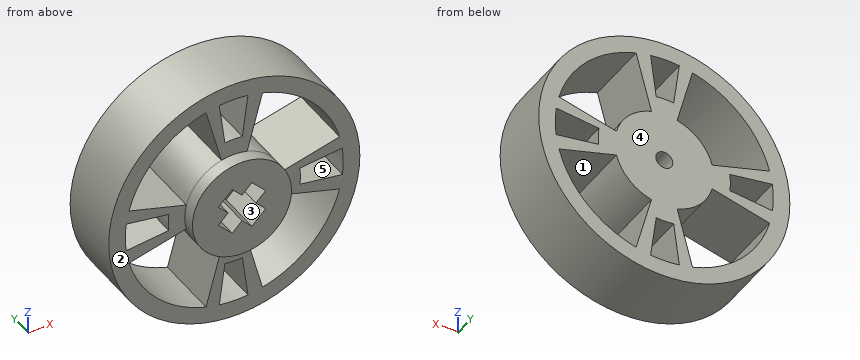
from build123d import *

# Parameters (mm, degrees)
SKETCH1_R           = 9.525
BOSS_EXTRUDE1_DEPTH = 2.54
SKETCH3_R           = 24.13
BOSS_EXTRUDE2_DEPTH = 12.7
CUT_EXTRUDE2_DEPTH  = 16.24
CUT_EXTRUDE3_DEPTH  = 8.466666667
SKETCH5_R           = 1.63195
CUT_EXTRUDE4_DEPTH  = 16.24


with BuildPart() as part:
    # Sketch1 → Boss-Extrude1 (new body)
    with BuildSketch(Plane(origin=(0, 0, 0), x_dir=(1, 0, 0), z_dir=(0, 1, 0))):
        Circle(SKETCH1_R)
    extrude(amount=BOSS_EXTRUDE1_DEPTH)

    # Sketch3 → Boss-Extrude2 (add)
    with BuildSketch(Plane(origin=(0, 2.54, 0), x_dir=(1, 0, 0), z_dir=(0, 1, 0))):
        Circle(SKETCH3_R)
        with BuildLine():
            Line((-2.465251405, 9.200443495), (-5.42355309, 20.24097569))
            ThreePointArc((-5.42355309, 20.24097569), (-14.8174226, 14.8174226), (-20.24097569, 5.42355309))
            Line((-20.24097569, 5.42355309), (-9.200443495, 2.465251405))
            ThreePointArc((-9.200443495, 2.465251405), (-6.735192091, 6.735192091), (-2.465251405, 9.200443495))
        make_face(mode=Mode.SUBTRACT)
        with BuildLine():
            Line((9.200443495, 2.465251405), (20.24097569, 5.42355309))
            ThreePointArc((20.24097569, 5.42355309), (14.8174226, 14.8174226), (5.42355309, 20.24097569))
            Line((5.42355309, 20.24097569), (2.465251405, 9.200443495))
            ThreePointArc((2.465251405, 9.200443495), (6.735192091, 6.735192091), (9.200443495, 2.465251405))
        make_face(mode=Mode.SUBTRACT)
        with BuildLine():
            Line((9.200443495, -2.465251405), (20.24097569, -5.42355309))
            ThreePointArc((20.24097569, -5.42355309), (14.8174226, -14.8174226), (5.42355309, -20.24097569))
            Line((5.42355309, -20.24097569), (2.465251405, -9.200443495))
            ThreePointArc((2.465251405, -9.200443495), (6.735192091, -6.735192091), (9.200443495, -2.465251405))
        make_face(mode=Mode.SUBTRACT)
        with BuildLine():
            Line((-9.200443495, -2.465251405), (-20.24097569, -5.42355309))
            ThreePointArc((-20.24097569, -5.42355309), (-14.8174226, -14.8174226), (-5.42355309, -20.24097569))
            Line((-5.42355309, -20.24097569), (-2.465251405, -9.200443495))
            ThreePointArc((-2.465251405, -9.200443495), (-6.735192091, -6.735192091), (-9.200443495, -2.465251405))
        make_face(mode=Mode.SUBTRACT)
    extrude(amount=BOSS_EXTRUDE2_DEPTH)

    # Sketch4 → Cut-Extrude2 (cut, through all)
    with BuildSketch(Plane(origin=(0, 15.24, 0), x_dir=(1, 0, 0), z_dir=(0, 1, 0))):
        with BuildLine():
            Line((12.604555768, 1.554082971), (20.78910082, 2.631598769))
            ThreePointArc((20.78910082, 2.631598769), (20.95460619, -0.128469511), (20.755271414, -2.886301011))
            Line((20.755271414, -2.886301011), (12.570536445, -1.80876021))
            ThreePointArc((12.570536445, -1.80876021), (12.699350202, -0.128469656), (12.604555768, 1.554082971))
        make_face()
        with BuildLine():
            Line((-12.604555768, 1.554082971), (-20.78910082, 2.631598769))
            ThreePointArc((-20.78910082, 2.631598769), (-20.95460619, -0.128469511), (-20.755271414, -2.886301011))
            Line((-20.755271414, -2.886301011), (-12.570536445, -1.80876021))
            ThreePointArc((-12.570536445, -1.80876021), (-12.699350202, -0.128469656), (-12.604555768, 1.554082971))
        make_face()
        with BuildLine():
            Line((1.554082971, 12.604555768), (2.631598769, 20.78910082))
            ThreePointArc((2.631598769, 20.78910082), (-0.128469511, 20.95460619), (-2.886301011, 20.755271414))
            Line((-2.886301011, 20.755271414), (-1.80876021, 12.570536445))
            ThreePointArc((-1.80876021, 12.570536445), (-0.128469656, 12.699350202), (1.554082971, 12.604555768))
        make_face()
        with BuildLine():
            Line((-1.80876021, -12.570536445), (-2.886301011, -20.755271414))
            ThreePointArc((-2.886301011, -20.755271414), (-0.128469511, -20.95460619), (2.631598769, -20.78910082))
            Line((2.631598769, -20.78910082), (1.554082971, -12.604555768))
            ThreePointArc((1.554082971, -12.604555768), (-0.128469656, -12.699350202), (-1.80876021, -12.570536445))
        make_face()
    extrude(amount=-CUT_EXTRUDE2_DEPTH, mode=Mode.SUBTRACT)

    # Sketch2 → Cut-Extrude3 (cut)
    with BuildSketch(Plane(origin=(0, 0, 0), x_dir=(1, 0, 0), z_dir=(0, 1, 0))):
        Polygon((-4.552853785, 1.885853785), (-1.885853785, 4.552853785), (0, 2.667), (1.885853785, 4.552853785), (4.552853785, 1.885853785), (2.667, 0), (4.552853785, -1.885853785), (1.885853785, -4.552853785), (0, -2.667), (-1.885853785, -4.552853785), (-4.552853785, -1.885853785), (-2.667, 0), align=None)
    extrude(amount=CUT_EXTRUDE3_DEPTH, mode=Mode.SUBTRACT)

    # Sketch5 → Cut-Extrude4 (cut, through all)
    with BuildSketch(Plane(origin=(0, 15.24, 0), x_dir=(1, 0, 0), z_dir=(0, 1, 0))):
        Circle(SKETCH5_R)
    extrude(amount=-CUT_EXTRUDE4_DEPTH, mode=Mode.SUBTRACT)


solid = part.part
Model file for the job. Use its own axes, mm. Face numbers are marked on the shaded views. A direction names the side the tool comes from. Give positions to 0.01 mm unless a question says otherwise; leave off trailing zeros. Loops run counter-clockwise (first coordinate to the right, second up) from the corner with the lowest first, then second, coordinate; pieces in that order, holes last.
Item 1: Slice it at D-D (z = 8). Write the cut outline in (x, y).
Check values:
outline: (-22.77, 2.54) - (-19.37, 2.54) - (-19.37, 15.24) - (-22.77, 15.24) - close; (-5.17, 0) - (5.17, 0) - (5.17, 15.24) - (-5.17, 15.24) - close; (19.37, 2.54) - (22.77, 2.54) - (22.77, 15.24) - (19.37, 15.24) - close
Item 2: Slice it at A-A (y = 13.5). Give the number of separate pieces and of enclosed holes in the cut face, plus the area to 3 significant figures.
Check values:
separate pieces: 1
enclosed holes: 9
area: 944 mm2
Item 3: Mould opens along X. For the marked faces 1 and 2 say: +X half, -X half, draft (parallel to the pull), parting line (faces both ways), or undercut.
Check values:
face 1: undercut
face 2: draft
Item 4: Slice it at C-C (x = 18). Write the cut outline in (y, z), plus the area to 3 significant figures.
Check values:
outline: (2.54, -16.07) - (15.24, -16.07) - (15.24, -10.73) - (2.54, -10.73) - close; (2.54, -4.82) - (15.24, -4.82) - (15.24, -2.26) - (2.54, -2.26) - close; (2.54, 2.52) - (15.24, 2.52) - (15.24, 4.82) - (2.54, 4.82) - close; (2.54, 10.73) - (15.24, 10.73) - (15.24, 16.07) - (2.54, 16.07) - close
area: 197 mm2
Item 5: Which spindle directions (+Z, -Z, +X, -X, +Y, -Y) get a long thin tool onto all of the face, cutting with end or side? Do the marked faces 3, 4 and 5. Say none if no direction does.
Check values:
face 3: -Y
face 4: +Z, -Z, +X, -X, +Y
face 5: +Y, -Y
Item 6: Slice it at B-B (z = 1). Write the cut outline in (x, y), plus the area to 3 significant figures.
Check values:
outline: (-24.11, 2.54) - (-20.93, 2.54) - (-20.93, 15.24) - (-24.11, 15.24) - close; (-12.66, 2.54) - (-9.47, 2.54) - (-9.47, 0) - (-3.67, 0) - (-3.67, 8.47) - (-1.29, 8.47) - (-1.29, 15.24) - (-12.66, 15.24) - close; (1.29, 8.47) - (3.67, 8.47) - (3.67, 0) - (9.47, 0) - (9.47, 2.54) - (12.66, 2.54) - (12.66, 15.24) - (1.29, 15.24) - close; (20.93, 2.54) - (24.11, 2.54) - (24.11, 15.24) - (20.93, 15.24) - close
area: 371 mm2
Item 7: Drop flat-ended pins along their axis: P1, Ø10, axis at x = 5.5, z = -17, coming from the -Y side; P2, Ø5, axis at y = 7, z = 7.5, coming from the -X side; P3, Ø8, axis at y = 9.5, z = -7.5, coming from the +X side. Give the stop position or say it passes through.
Check values:
P1: stops at y = 2.54
P2: stops at x = -23.61
P3: stops at x = 23.87
Item 8: Drill centre lines: line 1 along Z through (x, y) = (0, 13.25) (3 decimals); line 2 along Z through (x, y) = (-18, 14). Where is each one in solid material? Low to high.
Check values:
line 1: z = -24.13 to -20.955, -12.7 to -1.632, 1.632 to 12.7, 20.955 to 24.13
line 2: z = -16.07 to -10.73, -4.82 to -2.26, 2.52 to 4.82, 10.73 to 16.07
